from build123d import *

# Parameters (mm, degrees)
ESQUISSE1_W             = 17
ESQUISSE1_H             = 20
BOSS_EXTRU_1_DEPTH      = 19.5
ESQUISSE2_R             = 3.175
ENL_V_MAT_EXTRU_1_DEPTH = 18
ESQUISSE3_R             = 3.175
ENL_V_MAT_EXTRU_2_DEPTH = 12.7
ESQUISSE4_R             = 1.35255
ENL_V_MAT_EXTRU_3_DEPTH = 18


with BuildPart() as part:
    # Esquisse1 → Boss.-Extru.1 (new body, symmetric)
    with BuildSketch(Plane(origin=(0, 0, 0), x_dir=(1, 0, 0), z_dir=(0, 1, 0))):
        Rectangle(ESQUISSE1_W, ESQUISSE1_H)
    extrude(amount=BOSS_EXTRU_1_DEPTH, both=True)

    # Esquisse2 → Enlèv. mat.-Extru.1 (cut, through all)
    with BuildSketch(Plane.ZY.offset(8.5)):
        with Locations((0, -9.34)):
            Circle(ESQUISSE2_R)
    extrude(amount=-ENL_V_MAT_EXTRU_1_DEPTH, mode=Mode.SUBTRACT)

    # Esquisse3 → Enlèv. mat.-Extru.2 (cut)
    with BuildSketch(Plane(origin=(0, 19.5, 0), x_dir=(1, 0, 0), z_dir=(0, 1, 0))):
        Circle(ESQUISSE3_R)
    extrude(amount=-ENL_V_MAT_EXTRU_2_DEPTH, mode=Mode.SUBTRACT)

    # Esquisse4 → Enlèv. mat.-Extru.3 (cut, through all)
    with BuildSketch(Plane(origin=(8.5, 0, 0), x_dir=(0, 0, -1), z_dir=(1, 0, 0))):
        with Locations((-6.914797213, -2.425202787)):
            Circle(ESQUISSE4_R)
        with Locations((6.914797213, -2.425202787)):
            Circle(ESQUISSE4_R)
        with Locations((-6.914797213, -16.254797213)):
            Circle(ESQUISSE4_R)
        with Locations((6.914797213, -16.254797213)):
            Circle(ESQUISSE4_R)
    extrude(amount=-ENL_V_MAT_EXTRU_3_DEPTH, mode=Mode.SUBTRACT)


solid = part.part
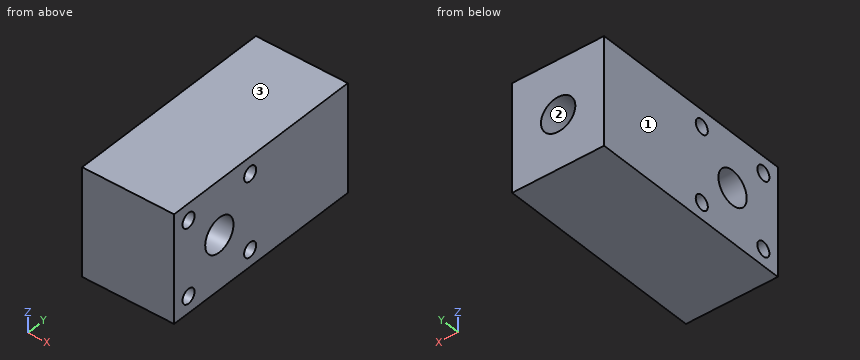
Work out the finished part from the listing and answer in its coordinate system (mm). Face numbers are marked on the shaded views. Round coordinates to 2 decimals unless told otherwise and drop trailing zeros. Write each loop counter-clockwise with the first axis right and the second up, starting at its lowest first coordinate (ties: lowest second). Pieces come first, ordered by that corner, then holes. Notation, with made-up numbers: M 56,53.5 L 60,53.5 A13 cw 60,72.5 Z; hole C 39.5,55.5 d2. An arc over 180 degrees is marked long. Use a Markdown table: item, result.
1) The part is cut by section D-D on z = 7.75. Give the vertices of the cut face in (x, y).
Taken from the geometry:
| item | result |
|---|---|
| outline | M -8.5,-19.5 L 8.5,-19.5 L 8.5,-17.32 L -8.5,-17.32 Z; M -8.5,-15.19 L 8.5,-15.19 L 8.5,-3.49 L -8.5,-3.49 Z; M -8.5,-1.36 L 8.5,-1.36 L 8.5,19.5 L -8.5,19.5 Z |
2) Determine the mould class of the marked faces 1, 2 and 3 for opening direction Z: pulls with the +Z half, pulls with the -Z half, needs draft (parallel to the pull), parting line crosses it, or undercut.
Taken from the geometry:
| item | result |
|---|---|
| face 1 | needs draft |
| face 2 | undercut |
| face 3 | pulls with the +Z half |
3) The part is cut by section B-B on z = 0.5. Give the vertices of the cut face in (x, y).
Taken from the geometry:
| item | result |
|---|---|
| outline | M -8.5,-19.5 L 8.5,-19.5 L 8.5,-12.48 L -8.5,-12.48 Z; M -8.5,-6.2 L 8.5,-6.2 L 8.5,19.5 L 3.14,19.5 L 3.14,6.8 L -3.14,6.8 L -3.14,19.5 L -8.5,19.5 Z |
4) Flat-ended cylindrical pins translate along their axes: pin 1 (5 mm diameter, centred on y = -9.34, z = 0, fed in from -X); pin 2 (5 mm diameter, centred on x = 0, z = 0, fed in from +Y). Find the tip coordinate at first contact, or state that the pin passes through.
Taken from the geometry:
| item | result |
|---|---|
| pin 1 | passes through |
| pin 2 | stops at y = 6.8 |
5) Consider line 1 (Y direction, x = -3.25, z = -6.75); line 2 (Z direction, x = 2.25, y = -15.5); line 3 (X direction, y = 14.5, z = 0) (3 decimals). Determine where each line is inside the solid, lowest interval first. Write a range as [from, to].
Taken from the geometry:
| item | result |
|---|---|
| line 1 | y = [-19.5, -17.6], [-14.91, -3.77], [-1.08, 19.5] |
| line 2 | z = [-10, -8.04], [-5.79, 5.79], [8.04, 10] |
| line 3 | x = [-8.5, -3.175], [3.175, 8.5] |
6) The part is cut by section A-A on y = -9.34. Give the vertices of the cut face in (x, z) (3 decimals).
Taken from the geometry:
| item | result |
|---|---|
| outline | M -8.5,-10 L 8.5,-10 L 8.5,-3.175 L -8.5,-3.175 Z; M -8.5,3.175 L 8.5,3.175 L 8.5,10 L -8.5,10 Z |
7) The part is cut by section C-C on x = -6.5. Give the vertices of the cut face in (y, z) (3 decimals).
Taken from the geometry:
| item | result |
|---|---|
| outline | M -19.5,-10 L 19.5,-10 L 19.5,10 L -19.5,10 Z; hole C -16.255,-6.915 d2.705; hole C -16.255,6.915 d2.705; hole C -9.34,0 d6.35; hole C -2.425,-6.915 d2.705; hole C -2.425,6.915 d2.705 |
